Design review of the part built by this model. Coordinates are the model's own, in mm. Face numbers are marked on the shaded views. Coordinates: 2 decimals unless noted, no trailing zeros. Loops run counter-clockwise (first coordinate to the right, second up) from the corner with the lowest first, then second, coordinate; pieces in that order, holes last. Notation, with made-up numbers: (0, 11.5) - (47, 11.5) arc R20 cw to (47, 42.5) - close; hole circle Ø4 at (57.5, -26.75). An arc over 180 degrees is marked (long way). Use one line per item in the form item = value. Start each with the question number.
(1) Add section B-B (z = -25.4). State the section outline as (x, y) points, plus the area to 3 significant figures.
(2) Add section C-C (y = 4). State the section outline as (x, z) points.
(3) The part is to be moulded in two halves that separate along Z. For the marked faces 1, 2, 3 and 4, say which applies: pulls with the +Z half, pulls with the -Z half, needs draft (parallel to the pull), parting line crosses it, or undercut.
(4) Clearance check with flat-ended pins moving along their axes: pin 1 Ø2 at (y, z) = (5, -24.5) entering from +X; pin 2 Ø1.5 at (y, z) = (9.5, -9.5) entering from +X. State where each tip first meets the part, or that it passes through.
(5) Add section D-D (x = 39.5). State the section outline as (y, z) points, plus the area to 3 significant figures.
(6) For L1, parallel to Y at x = 4, z = -25; L2, parallel to Y at x = 1.5, z = -25.4; L3, parallel to X at y = 22, z = -36, list the stretches that pass through material, from the lowest coordinate up.
(7) Add section A-A (y = 12.7). State the section outline as (x, z) points.
```python
from build123d import *

# Parameters (mm, degrees)
SKETCH1_W           = 6.35
SKETCH1_H           = 38.1
SKETCH1_H_2         = 6.35
SKETCH1_W_2         = 76.2
BOSS_EXTRUDE1_DEPTH = 25.4
SKETCH2_R           = 3.302
CUT_EXTRUDE1_DEPTH  = 7.35
SKETCH3_R           = 4.7625
CUT_EXTRUDE2_DEPTH  = 7.35
FILLET1_R           = 2.54


with BuildPart() as part:
    # Sketch1 → Boss-Extrude1 (new body)
    with BuildSketch(Plane(origin=(0, 0, 0), x_dir=(1, 0, 0), z_dir=(0, 1, 0))):
        with Locations((3.175, 25.4)):
            Rectangle(SKETCH1_W, SKETCH1_H)
        with Locations((3.175, 3.175)):
            Rectangle(SKETCH1_W, SKETCH1_H_2)
        with Locations((44.45, 3.175)):
            Rectangle(SKETCH1_W_2, SKETCH1_H_2)
    extrude(amount=BOSS_EXTRUDE1_DEPTH)

    # Sketch2 → Cut-Extrude1 (cut, through all)
    with BuildSketch(Plane(origin=(0, 0, -6.35), x_dir=(-1, 0, 0), z_dir=(0, 0, -1))):
        with Locations((-73.025, 12.7)):
            Circle(SKETCH2_R)
    extrude(amount=-CUT_EXTRUDE1_DEPTH, mode=Mode.SUBTRACT)

    # Sketch3 → Cut-Extrude2 (cut, through all)
    with BuildSketch(Plane(origin=(6.35, 0, 0), x_dir=(0, 0, -1), z_dir=(1, 0, 0))):
        with Locations((25.4, 12.7)):
            Circle(SKETCH3_R)
    extrude(amount=-CUT_EXTRUDE2_DEPTH, mode=Mode.SUBTRACT)

    # Fillet1
    fillet1_edges = [part.edges().sort_by_distance(p)[0] for p in [
        (0, 12.7, -44.45),
        (6.35, 12.7, -44.45),
        (6.35, 12.7, -6.35),
        (82.55, 12.7, -6.35),
        (82.55, 12.7, 0),
        (0, 12.7, 0),
    ]]
    fillet(fillet1_edges, radius=FILLET1_R)


solid = part.part
```
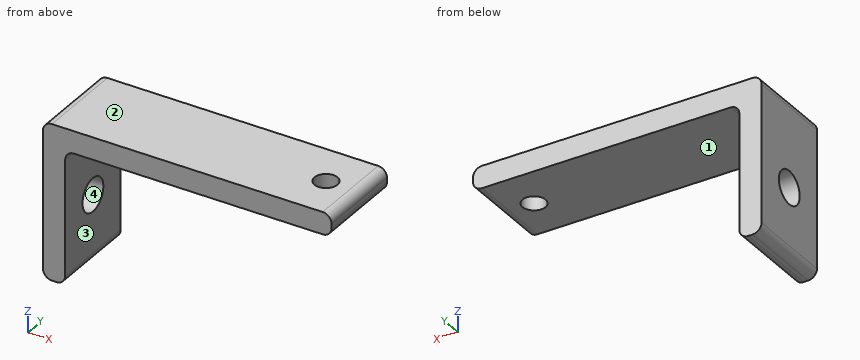
Computed values:
q1.outline = (0, 0) - (6.35, 0) - (6.35, 7.94) - (0, 7.94) - close; (0, 17.46) - (6.35, 17.46) - (6.35, 25.4) - (0, 25.4) - close
q1.area = 101 mm^2
q2.outline = (0, -41.91) arc R2.54 ccw to (2.54, -44.45) - (3.81, -44.45) arc R2.54 ccw to (6.35, -41.91) - (6.35, -8.89) arc R2.54 cw to (8.89, -6.35) - (80.01, -6.35) arc R2.54 ccw to (82.55, -3.81) - (82.55, -2.54) arc R2.54 ccw to (80.01, 0) - (2.54, 0) arc R2.54 ccw to (0, -2.54) - close
q3.face_1 = pulls with the -Z half
q3.face_2 = pulls with the +Z half
q3.face_3 = needs draft
q3.face_4 = undercut
q4.pin_1 = 6.35
q4.pin_2 = 6.35
q5.outline = (0, -6.35) - (25.4, -6.35) - (25.4, 0) - (0, 0) - close
q5.area = 161 mm^2
q6.L1 = 0 to 7.95, 17.45 to 25.4
q6.L2 = 0 to 7.94, 17.46 to 25.4
q6.L3 = 0 to 6.35
q7.outline = (0, -41.91) arc R2.54 ccw to (2.54, -44.45) - (3.81, -44.45) arc R2.54 ccw to (6.35, -41.91) - (6.35, -30.16) - (0, -30.16) - close; (0, -20.64) - (6.35, -20.64) - (6.35, -8.89) arc R2.54 cw to (8.89, -6.35) - (69.72, -6.35) - (69.72, 0) - (2.54, 0) arc R2.54 ccw to (0, -2.54) - close; (76.33, -6.35) - (80.01, -6.35) arc R2.54 ccw to (82.55, -3.81) - (82.55, -2.54) arc R2.54 ccw to (80.01, 0) - (76.33, 0) - close
